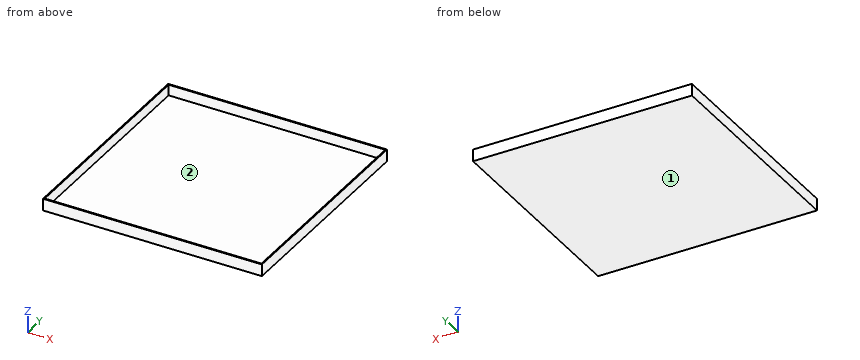
```python
from build123d import *

# Parameters (mm, degrees)
SKETCH_2_W      = 202
SKETCH_2_H      = 202
EXTRUDE_1_DEPTH = 11
SKETCH_1_W      = 200
SKETCH_1_H      = 200
EXTRUDE_2_DEPTH = 10


with BuildPart() as part:
    # 草图2 → 凸台-拉伸1 (new body)
    with BuildSketch(Plane.XY):
        with Locations((86.004694039, 88.571428571)):
            Rectangle(SKETCH_2_W, SKETCH_2_H)
    extrude(amount=-EXTRUDE_1_DEPTH)


with BuildPart() as body_2:
    # 草图1 → 凸台-拉伸2 (new body)
    with BuildSketch(Plane.XY):
        with Locations((86.004694039, 88.571428571)):
            Rectangle(SKETCH_1_W, SKETCH_1_H)
    extrude(amount=-EXTRUDE_2_DEPTH)


with BuildPart() as part_1:
    add(part.part)

    # Combine 1: cut body 2
    add(body_2.part, mode=Mode.SUBTRACT)


solid = part_1.part
```
Source: CAD feature listing. Evaluate the final solid. Frame: model axes, mm. Face numbers are marked on the shaded views. Round coordinates to 2 decimals unless told otherwise and drop trailing zeros. Loops run counter-clockwise (first coordinate to the right, second up) from the corner with the lowest first, then second, coordinate; pieces in that order, holes last. Notation, with made-up numbers: M 6.5,57.25 L 32.5,57.25 A17 ccw 32.5,75.25 Z; hole C 72.5,10.5 d2. An arc over 180 degrees is marked long. Put each result on its own line as item: value.
(1) Pull-direction query (X, two-part tool) for the marked faces 1 and 2; classes: released by +X, released by -X, zero draft, split by the parting line, or undercut.
Solutions:
face 1: zero draft
face 2: undercut
(2) Ray query, line 1 (X direction, y = 13.5, z = -9); line 2 (Y direction, x = 105.5, z = -4); line 3 (Z direction, x = 20.5, y = 160). Return the intervals inside material, ascending. Write a range as [from, to].
Solutions:
line 1: [-15, -14], [186, 187]
line 2: [-12.43, -11.43], [188.57, 189.57]
line 3: [-11, -10]
(3) First-contact query: pin 1 (1 mm diameter, centred on x = 62, y = 126.5, fed in from +Z). Flat tip, straight axial feed; report the tip coordinate or a pass-through.
Solutions:
pin 1: z = -10
(4) Section B-B, the plane x = 98.5. Return loops of the section in (y, z).
Solutions:
outline: M -12.43,-11 L 189.57,-11 L 189.57,0 L 188.57,0 L 188.57,-10 L -11.43,-10 L -11.43,0 L -12.43,0 Z
(5) Section C-C, the plane y = 176. Return loops of the section in (x, z).
Solutions:
outline: M -15,-11 L 187,-11 L 187,0 L 186,0 L 186,-10 L -14,-10 L -14,0 L -15,0 Z
(6) Section A-A, the plane z = -2.5. Return loops of the section in (x, y), and give its area (3 significant figures).
Solutions:
outline: M -15,-12.43 L 187,-12.43 L 187,189.57 L -15,189.57 Z; hole M -14,-11.43 L 186,-11.43 L 186,188.57 L -14,188.57 Z
area: 804 mm²
